```python
from build123d import *

# Parameters (mm, degrees)
F0_W            = 48
F0_H            = 48
F1_DEPTH        = 48
F2_R            = 1
F3_R            = 1
F4_T1_DEPTH     = 46
F4_T3_DEPTH     = 46
F4_T5_DEPTH     = 46
F4_S9_W         = 1
F4_S9_H         = 1
F4_T10_DEPTH    = 1
F4_S15_W        = 1
F4_S15_H        = 1
F4_T16_DEPTH    = 1
F4_S21_W        = 1
F4_S21_H        = 1
F4_T22_DEPTH    = 1
F4_S27_W        = 1
F4_S27_H        = 1
F4_T28_DEPTH    = 1
F4_T32_ANGLE    = 90
F4_T34_ANGLE    = 90
F6_D            = 18
F6_CSINK_D      = 36
F6_CSINK_ANGLE  = 90
F8_D            = 18
F8_CSINK_D      = 36
F8_CSINK_ANGLE  = 90
F10_D           = 18
F10_CSINK_D     = 36
F10_CSINK_ANGLE = 90


# Not quite as in the source:
# - a fillet or chamfer that OpenCascade refuses, or shapes differently, is made with other operations: its cross-section is extruded or revolved along the edge and cut away or added


with BuildPart() as f1:
    # F0 (on Front) → F1 (new body)
    with BuildSketch(Plane.XZ):
        Rectangle(F0_W, F0_H)
    extrude(amount=F1_DEPTH)

    # F2
    f2_edges = [f1.edges().sort_by_distance(p)[0] for p in [
        (24, -24, 24),
    ]]
    fillet(f2_edges, radius=F2_R)

    # F3
    f3_edges = [f1.edges().sort_by_distance(p)[0] for p in [
        (-24, -24, 24),
        (-0.5, 0, 24),
        (-0.5, -48, 24),
    ]]
    fillet(f3_edges, radius=F3_R)

    # F4: fillet of radius 1 on 8 edges, made by hand

    # F4_s2 → F4_t1 (cut)
    with BuildSketch(Plane.XY.offset(-23)):
        with BuildLine():
            ThreePointArc((-23, -48), (-23.7071067812, -47.7071067812), (-24, -47))
            Line((-24, -47), (-24, -48))
            Line((-24, -48), (-23, -48))
        make_face()
        with BuildLine():
            ThreePointArc((-23, 0), (-23.7071067812, -0.2928932188), (-24, -1))
            Line((-24, -1), (-24, 0))
            Line((-24, 0), (-23, 0))
        make_face()
    extrude(amount=F4_T1_DEPTH, mode=Mode.SUBTRACT)

    # F4_s4 → F4_t3 (cut)
    with BuildSketch(Plane.YZ.offset(-23)):
        with BuildLine():
            ThreePointArc((0, -23), (-0.2928932188, -23.7071067812), (-1, -24))
            Line((-1, -24), (0, -24))
            Line((0, -24), (0, -23))
        make_face()
        with BuildLine():
            ThreePointArc((-48, -23), (-47.7071067812, -23.7071067812), (-47, -24))
            Line((-47, -24), (-48, -24))
            Line((-48, -24), (-48, -23))
        make_face()
    extrude(amount=F4_T3_DEPTH, mode=Mode.SUBTRACT)

    # F4_s6 → F4_t5 (cut)
    with BuildSketch(Plane.XZ.offset(1)):
        with BuildLine():
            ThreePointArc((-24, -23), (-23.7071067812, -23.7071067812), (-23, -24))
            Line((-23, -24), (-24, -24))
            Line((-24, -24), (-24, -23))
        make_face()
        with BuildLine():
            ThreePointArc((24, -23), (23.7071067812, -23.7071067812), (23, -24))
            Line((23, -24), (24, -24))
            Line((24, -24), (24, -23))
        make_face()
    extrude(amount=F4_T5_DEPTH, mode=Mode.SUBTRACT)


with BuildPart() as f4_tool8:
    # F4_s9 → F4_t10 (new body)
    with BuildSketch(Plane.XZ.offset(1)):
        with Locations((-23.5, 23.5)):
            Rectangle(F4_S9_W, F4_S9_H)
    extrude(amount=-F4_T10_DEPTH)

    # F4_s11 → F4_t12 (revolve, cut)
    with BuildSketch(Plane(origin=(-23, -1, 23), x_dir=(0.7071067812, 0, -0.7071067812), z_dir=(0.7071067812, 0, 0.7071067812))):
        with BuildLine():
            ThreePointArc((0, -1), (1, 0), (0, 1))
            Line((0, 1), (0, -1))
        make_face()
    revolve(axis=Axis((-23, -1, 23), (0, 1, 0)), mode=Mode.SUBTRACT)


with BuildPart() as f1_1:
    add(f1.part)

    # F4_t7: cut F4_tool8
    add(f4_tool8.part, mode=Mode.SUBTRACT)


with BuildPart() as f4_tool14:
    # F4_s15 → F4_t16 (new body)
    with BuildSketch(Plane.XZ.offset(47)):
        with Locations((-23.5, 23.5)):
            Rectangle(F4_S15_W, F4_S15_H)
    extrude(amount=F4_T16_DEPTH)

    # F4_s17 → F4_t18 (revolve, cut)
    with BuildSketch(Plane(origin=(-23, -47, 23), x_dir=(0.7071067812, 0, -0.7071067812), z_dir=(-0.7071067812, 0, -0.7071067812))):
        with BuildLine():
            ThreePointArc((0, -1), (1, 0), (0, 1))
            Line((0, 1), (0, -1))
        make_face()
    revolve(axis=Axis((-23, -47, 23), (0, -1, 0)), mode=Mode.SUBTRACT)


with BuildPart() as f1_2:
    add(f1_1.part)

    # F4_t13: cut F4_tool14
    add(f4_tool14.part, mode=Mode.SUBTRACT)


with BuildPart() as f4_tool20:
    # F4_s21 → F4_t22 (new body)
    with BuildSketch(Plane.XZ.offset(47)):
        with Locations((-23.5, -23.5)):
            Rectangle(F4_S21_W, F4_S21_H)
    extrude(amount=F4_T22_DEPTH)

    # F4_s23 → F4_t24 (revolve, cut)
    with BuildSketch(Plane(origin=(-23, -47, -23), x_dir=(0.7071067812, 0, 0.7071067812), z_dir=(0.7071067812, 0, -0.7071067812))):
        with BuildLine():
            ThreePointArc((0, -1), (1, 0), (0, 1))
            Line((0, 1), (0, -1))
        make_face()
    revolve(axis=Axis((-23, -47, -23), (0, -1, 0)), mode=Mode.SUBTRACT)


with BuildPart() as f1_3:
    add(f1_2.part)

    # F4_t19: cut F4_tool20
    add(f4_tool20.part, mode=Mode.SUBTRACT)


with BuildPart() as f4_tool26:
    # F4_s27 → F4_t28 (new body)
    with BuildSketch(Plane.XZ.offset(1)):
        with Locations((-23.5, -23.5)):
            Rectangle(F4_S27_W, F4_S27_H)
    extrude(amount=-F4_T28_DEPTH)

    # F4_s29 → F4_t30 (revolve, cut)
    with BuildSketch(Plane(origin=(-23, -1, -23), x_dir=(0.7071067812, 0, 0.7071067812), z_dir=(-0.7071067812, 0, 0.7071067812))):
        with BuildLine():
            ThreePointArc((0, -1), (1, 0), (0, 1))
            Line((0, 1), (0, -1))
        make_face()
    revolve(axis=Axis((-23, -1, -23), (0, 1, 0)), mode=Mode.SUBTRACT)


with BuildPart() as f1_4:
    add(f1_3.part)

    # F4_t25: cut F4_tool26
    add(f4_tool26.part, mode=Mode.SUBTRACT)

    # F4_s31 → F4_t32 (revolve, cut)
    with BuildSketch(Plane.XZ.offset(1)):
        with BuildLine():
            ThreePointArc((24, -23), (23.7071067812, -23.7071067812), (23, -24))
            Line((23, -24), (24, -24))
            Line((24, -24), (24, -23))
        make_face()
    revolve(axis=Axis((23, -1, -24), (0, 0, 1)), revolution_arc=F4_T32_ANGLE, mode=Mode.SUBTRACT)

    # F4_s33 → F4_t34 (revolve, cut)
    with BuildSketch(Plane.XZ.offset(47)):
        with BuildLine():
            ThreePointArc((24, -23), (23.7071067812, -23.7071067812), (23, -24))
            Line((23, -24), (24, -24))
            Line((24, -24), (24, -23))
        make_face()
    revolve(axis=Axis((23, -47, -24), (0, 0, -1)), revolution_arc=F4_T34_ANGLE, mode=Mode.SUBTRACT)

    # F6 (through all)
    with Locations(Plane.XY.offset(24)):
        with Locations((0, -24)):
            CounterSinkHole(F6_D / 2, F6_CSINK_D / 2, counter_sink_angle=F6_CSINK_ANGLE)

    # F8 (through all)
    with Locations(Plane(origin=(-24, 0, 0), x_dir=(0, -1, 0), z_dir=(-1, 0, 0))):
        with Locations((24, 0)):
            CounterSinkHole(F8_D / 2, F8_CSINK_D / 2, counter_sink_angle=F8_CSINK_ANGLE)

    # F10 (through all)
    with Locations(Plane.XZ.offset(48)):
        with Locations((0, 0)):
            CounterSinkHole(F10_D / 2, F10_CSINK_D / 2, counter_sink_angle=F10_CSINK_ANGLE)


solid = f1_4.part
```
Input: part model. Units: mm. Frame: model coordinates. Coordinates: 2 decimals unless noted, no trailing zeros. Loops run counter-clockwise (first coordinate to the right, second up) from the corner with the lowest first, then second, coordinate; pieces in that order, holes last.
Q1. Section C-C, the plane x = 20. Return the cut outline in (y, z), and give its area (3 significant figures).
Results are:
outline: (-48, -23) arc R1 ccw to (-47, -24) - (-1, -24) arc R1 ccw to (0, -23) - (0, 23) arc R1 ccw to (-1, 24) - (-47, 24) arc R1 ccw to (-48, 23) - close; hole circle Ø18 at (-24, 0)
area: 2,050 mm2
Q2. Line query: line 1 along Z through (x, y) = (18.5, -24); line 2 along X through (y, z) = (-24, 11.25); line 3 along Y through (x, z) = (-22, -10). Output: solid intervals per line, ascending.
Results are:
line 1: z = -24 to -9, 9 to 24
line 2: x = -17.25 to -9, 9 to 24
line 3: y = -48 to -36.49, -11.51 to 0
Q3. Mould query, pull axis Z, two halves, no side actions, for faces 1 (the conical face through (-4.355, -39.437, -8.372)), 2 (the flat face through (-11, 0, 0)), 3 (the conical face through (1.23, -14.64, 15.44)). Classes: +Z half, -Z half, draft (parallel to the pull), parting line (faces both ways), or undercut.
Results are:
face 1: undercut
face 2: draft
face 3: +Z half
Q4. Contact query for a flat-ended pin moving along its axis: pin 1 (23.5 mm diameter, centred on x = 0, y = -24, fed in from +Z). Output: stop coordinate, or through.
Results are:
pin 1: stops at z = 17.75
Q5. Section A-A, the plane y = -24. Return the cut outline in (x, z), and give its area (3 significant figures).
Results are:
outline: (-24, -23) arc R1 ccw to (-23, -24) - (-9, -24) - (-9, -9) - (-15, -9) - (-24, -18) - close; (-24, 18) - (-15, 9) - (-9, 9) - (-9, 15) - (-18, 24) - (-23, 24) arc R1 ccw to (-24, 23) - close; (9, -24) - (23, -24) arc R1 ccw to (24, -23) - (24, -9) - (9, -9) - close; (9, 9) - (24, 9) - (24, 23) arc R1 ccw to (23, 24) - (18, 24) - (9, 15) - close
area: 737 mm2
Q6. Section B-B, the plane z = -21. Return the cut outline in (x, y), and give its area (3 significant figures).
Results are:
outline: (-24, -47) arc R1 ccw to (-23, -48) - (23, -48) arc R1 ccw to (24, -47) - (24, -1) arc R1 ccw to (23, 0) - (-23, 0) arc R1 ccw to (-24, -1) - close; hole circle Ø18 at (0, -24)
area: 2,050 mm2
Q7. Section D-D, the plane z = 0. Return the cut outline in (x, y).
Results are:
outline: (-24, -47) arc R1 ccw to (-23, -48) - (-18, -48) - (-9, -39) - (-9, -33) - (-15, -33) - (-24, -42) - close; (-24, -6) - (-15, -15) - (-9, -15) - (-9, 0) - (-23, 0) arc R1 ccw to (-24, -1) - close; (9, -39) - (18, -48) - (23, -48) arc R1 ccw to (24, -47) - (24, -33) - (9, -33) - close; (9, -15) - (24, -15) - (24, -1) arc R1 ccw to (23, 0) - (9, 0) - close
